Here's how the part is built. I have some questions about the finished solid (model axes, mm). Face numbers are marked on the shaded views. A direction names the side the tool comes from. Round coordinates to 2 decimals unless told otherwise and drop trailing zeros. Loops run counter-clockwise (first coordinate to the right, second up) from the corner with the lowest first, then second, coordinate; pieces in that order, holes last. Notation, with made-up numbers: (-29.5, 85) -> (10.5, 85) arc R27 ccw to (10.5, 114) -> close; hole circle Ø6 at (-29.5, 49). An arc over 180 degrees is marked (long way). Use one line per item in the form item = value. Start each with the question number.
Item 1: If we section it at A-A (x = 17.12): Write out the boundary of the cut face in (y, z).
Item 2: I'm going to push flat-ended pins straight in: pin 1 Ø0.8 at (x, y) = (18, -0.5) entering from -Z; pin 2 Ø0.5 at (x, z) = (4, 12.5) entering from -Y; pin 3 Ø0.8 at (y, z) = (-0.5, 12.5) entering from -X. Where does each tip first touch, or does it pass through?
Item 3: For the marked faces 1, 2 and 3, which set-ups out of +Z, -Z, +X, -X, +Y, -Y let a thin tool reach every point of the face, with its end or its side?
Item 4: If we section it at B-B (z = 1.3): State how many separate pieces and enclosed holes the cut face has, then the cut area to 3 significant figures.
Item 5: If we section it at C-C (z = 20.25): Write out the boundary of the cut face in (x, y), then the cut area to 3 significant figures.
Item 6: If I drill on L1, parallel to Z at x = 17.12, y = 0.5; L2, parallel to X at y = 2.5, z = 14.25; L3, parallel to Z at x = 10, y = 2, over which ranges is the centre line in solid material (lowest first)? Write a range as [from, to].
Item 7: If we section it at D-D (x = 8): Write out the boundary of the cut face in (y, z), then the cut area to 3 significant figures.
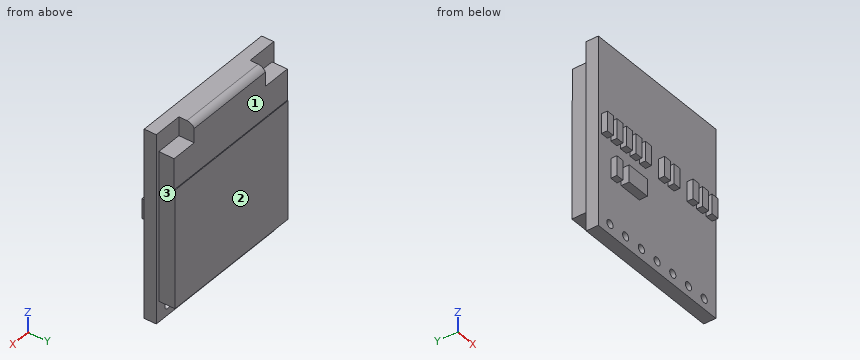
```python
from build123d import *

# Parameters (mm, degrees)
SKETCH1_W           = 19
SKETCH1_H           = 23.44
SKETCH1_R           = 0.5
BOSS_EXTRUDE1_DEPTH = 1.5
BOSS_EXTRUDE2_DEPTH = 2
FILLET1_R           = 1
SKETCH4_W           = 2.923966861
SKETCH4_H           = 2.115382352
BOSS_EXTRUDE3_DEPTH = 1
SKETCH5_W           = 0.965682683
SKETCH5_H           = 2.442516719
BOSS_EXTRUDE4_DEPTH = 0.75
CUT_EXTRUDE1_DEPTH  = 0.1


with BuildPart() as part:
    # Sketch1 → Boss-Extrude1 (new body)
    with BuildSketch(Plane(origin=(0, 0, 0), x_dir=(1, 0, 0), z_dir=(0, 1, 0))):
        with Locations((9.5, -11.72)):
            Rectangle(SKETCH1_W, SKETCH1_H)
        with Locations((1.88, -1.3)):
            Circle(SKETCH1_R, mode=Mode.SUBTRACT)
        with Locations((4.42, -1.3)):
            Circle(SKETCH1_R, mode=Mode.SUBTRACT)
        with Locations((6.96, -1.3)):
            Circle(SKETCH1_R, mode=Mode.SUBTRACT)
        with Locations((9.5, -1.3)):
            Circle(SKETCH1_R, mode=Mode.SUBTRACT)
        with Locations((12.04, -1.3)):
            Circle(SKETCH1_R, mode=Mode.SUBTRACT)
        with Locations((14.58, -1.3)):
            Circle(SKETCH1_R, mode=Mode.SUBTRACT)
        with Locations((17.12, -1.3)):
            Circle(SKETCH1_R, mode=Mode.SUBTRACT)
    extrude(amount=BOSS_EXTRUDE1_DEPTH)

    # Sketch3 → Boss-Extrude2 (add)
    with BuildSketch(Plane(origin=(0, 1.5, 0), x_dir=(1, 0, 0), z_dir=(0, 1, 0))):
        Polygon((3.832385917, -21.106985825), (3.832385917, -23.44), (15.344727023, -23.44), (15.344727023, -21.106985825), (18.591797592, -21.106985825), (18.591797592, -2.569164761), (0.290127115, -2.569164761), (0.290127115, -21.106985825), align=None)
    extrude(amount=BOSS_EXTRUDE2_DEPTH)

    # Fillet1
    fillet1_edges = [part.edges().sort_by_distance(p)[0] for p in [
        (9.58855647, 3.5, 23.44),
    ]]
    fillet(fillet1_edges, radius=FILLET1_R)

    # Sketch4 → Boss-Extrude3 (add)
    with BuildSketch(Plane.XZ):
        with Locations((5.157821851, 8.205990998)):
            Rectangle(SKETCH4_W, SKETCH4_H)
    extrude(amount=BOSS_EXTRUDE3_DEPTH)

    # Sketch5 → Boss-Extrude4 (add)
    with BuildSketch(Plane.XZ):
        with Locations((2.511251492, 12.877880521)):
            Rectangle(SKETCH5_W, SKETCH5_H)
        with Locations((0.971251492, 12.877880521)):
            Rectangle(SKETCH5_W, SKETCH5_H)
        with Locations((4.051251492, 12.877880521)):
            Rectangle(SKETCH5_W, SKETCH5_H)
        with Locations((5.591251492, 12.877880521)):
            Rectangle(SKETCH5_W, SKETCH5_H)
        with Locations((7.131251492, 12.877880521)):
            Rectangle(SKETCH5_W, SKETCH5_H)
        with Locations((10.211251492, 12.877880521)):
            Rectangle(SKETCH5_W, SKETCH5_H)
        with Locations((11.751251491, 12.877880521)):
            Rectangle(SKETCH5_W, SKETCH5_H)
        with Locations((14.831251492, 12.877880521)):
            Rectangle(SKETCH5_W, SKETCH5_H)
        with Locations((16.371251492, 12.877880521)):
            Rectangle(SKETCH5_W, SKETCH5_H)
        with Locations((17.911251492, 12.877880521)):
            Rectangle(SKETCH5_W, SKETCH5_H)
        with Locations((2.511251492, 8.277880522)):
            Rectangle(SKETCH5_W, SKETCH5_H)
    extrude(amount=BOSS_EXTRUDE4_DEPTH)

    # Sketch6 → Cut-Extrude1 (cut)
    with BuildSketch(Plane(origin=(0, 3.5, 0), x_dir=(1, 0, 0), z_dir=(0, 1, 0))):
        Polygon((0.290127115, -17.253788657), (18.591797592, -17.253788657), (18.591797592, -21.106985825), (15.344727023, -21.106985825), (15.344727023, -23.44), (3.832385917, -23.44), (3.832385917, -21.106985825), (0.290127115, -21.106985825), align=None)
    extrude(amount=-CUT_EXTRUDE1_DEPTH, mode=Mode.SUBTRACT)


solid = part.part
```
Values found:
q1.outline = (0, 0) -> (1.5, 0) -> (1.5, 0.8) -> (0, 0.8) -> close; (0, 1.8) -> (1.5, 1.8) -> (1.5, 2.57) -> (3.5, 2.57) -> (3.5, 17.25) -> (3.4, 17.25) -> (3.4, 21.11) -> (1.5, 21.11) -> (1.5, 23.44) -> (0, 23.44) -> close
q2.pin_1 = 11.66
q2.pin_2 = -0.75
q2.pin_3 = 0.49
q3.face_1 = +Z, +X, -X, +Y
q3.face_2 = +Z, -Z, +X, -X, +Y
q3.face_3 = +Z, -Z, +X, +Y
q4.separate_pieces = 8
q4.enclosed_holes = 0
q4.area = 18.0 mm2
q5.outline = (0, 0) -> (19, 0) -> (19, 1.5) -> (18.59, 1.5) -> (18.59, 3.4) -> (0.29, 3.4) -> (0.29, 1.5) -> (0, 1.5) -> close
q5.area = 63.3 mm2
q6.L1 = [0, 0.8], [1.8, 23.44]
q6.L2 = [0.29, 18.59]
q6.L3 = [2.57, 23.44]
q7.outline = (0, 0) -> (1.5, 0) -> (1.5, 2.57) -> (3.5, 2.57) -> (3.5, 17.25) -> (3.4, 17.25) -> (3.4, 22.88) arc R1 ccw to (2.5, 23.44) -> (0, 23.44) -> close
q7.area = 76.1 mm2
